The model under review builds one solid part; all positions refer to its coordinate system, in mm. Coordinates: 2 decimals unless noted, no trailing zeros. Write each loop counter-clockwise with the first axis right and the second up, starting at its lowest first coordinate (ties: lowest second). Pieces come first, ordered by that corner, then holes. Notation, with made-up numbers: (-29.5, -1.5) - (-17.5, -1.5) arc R10 cw to (-17.5, 5.5) - close; hole circle Ø6 at (67, 49). An arc over 180 degrees is marked (long way). Use one line per item in the form item = value. Start each with the question number.
```python
from build123d import *

# Parameters (mm, degrees)
SKETCH1_R           = 1.6
SKETCH1_R_2         = 3
BOSS_EXTRUDE1_DEPTH = 4
SKETCH2_R           = 11.550203763
CUT_EXTRUDE1_DEPTH  = 5


with BuildPart() as part:
    # Sketch1 → Boss-Extrude1 (new body)
    with BuildSketch(Plane.XY):
        with BuildLine():
            Line((27.071068699, -55.594908829), (62.571068699, -55.594908829))
            Line((62.571068699, -55.594908829), (62.571068699, -100.594908829))
            Line((62.571068699, -100.594908829), (24.071068699, -100.594908829))
            Line((24.071068699, -100.594908829), (24.071068699, -58.594908829))
            ThreePointArc((24.071068699, -58.594908829), (24.949748355, -56.473588486), (27.071068699, -55.594908829))
        make_face()
        with Locations((28.571068699, -64.094908829)):
            Circle(SKETCH1_R, mode=Mode.SUBTRACT)
        with Locations((44.071068699, -79.594908829)):
            Circle(SKETCH1_R_2, mode=Mode.SUBTRACT)
        with Locations((59.571068699, -64.094908829)):
            Circle(SKETCH1_R, mode=Mode.SUBTRACT)
        with Locations((28.571068699, -95.094908829)):
            Circle(SKETCH1_R, mode=Mode.SUBTRACT)
        with Locations((59.571068699, -95.094908829)):
            Circle(SKETCH1_R, mode=Mode.SUBTRACT)
    extrude(amount=BOSS_EXTRUDE1_DEPTH)

    # Sketch2 → Cut-Extrude1 (cut)
    with BuildSketch(Plane(origin=(0, 0, 0), x_dir=(-1, 0, 0), z_dir=(0, 0, -1))):
        with Locations((-44.071068699, -79.594908829)):
            Circle(SKETCH2_R)
    extrude(amount=-CUT_EXTRUDE1_DEPTH, mode=Mode.SUBTRACT)


solid = part.part
```
1. Take a section at B-B (x = 40.5). State the section outline as (y, z) points.
2. Take a section at A-A (y = -84.5). State the section outline as (x, z) points, plus the area to 3 significant figures.
3. Take a section at D-D (x = 60.5). State the section outline as (y, z) points, plus the area to 3 significant figures.
4. For L1, parallel to X at y = -64, z = 3.6; L2, parallel to Y at x = 44, z = 3.75; L3, parallel to Y at x = 44.5, z = 0.75, list the stretches that pass through material, from the lowest coordinate up.
5. The part is to be moulded in two halves that separate along X. For faces 1 (the cylindrical face through (24.927, -56.497, 1.972)), 2 (the cylindrical face through (38.74, -89.84, 1.97)), 3 (the cylindrical face through (58.392, -94.014, 1.972)), 4 (the flat face through (45, -55.595, 2)), say which applies: released by +X, released by -X, zero draft, split by the parting line, or undercut.
6. Take a section at C-C (z = 0.8). State the section outline as (x, y) points.
Returned:
q1.outline = (-100.59, 0) - (-90.58, 0) - (-90.58, 4) - (-100.59, 4) - close; (-68.61, 0) - (-55.59, 0) - (-55.59, 4) - (-68.61, 4) - close
q2.outline = (24.07, 0) - (33.61, 0) - (33.61, 4) - (24.07, 4) - close; (54.53, 0) - (62.57, 0) - (62.57, 4) - (54.53, 4) - close
q2.area = 70.3 mm²
q3.outline = (-100.59, 0) - (-96.4, 0) - (-96.4, 4) - (-100.59, 4) - close; (-93.79, 0) - (-65.4, 0) - (-65.4, 4) - (-93.79, 4) - close; (-62.79, 0) - (-55.59, 0) - (-55.59, 4) - (-62.79, 4) - close
q3.area = 159 mm²
q4.L1 = 24.07 to 26.97, 30.17 to 57.97, 61.17 to 62.57
q4.L2 = -100.59 to -91.14, -68.04 to -55.59
q4.L3 = -100.59 to -91.14, -68.05 to -55.59
q5.face_1 = released by -X
q5.face_2 = undercut
q5.face_3 = undercut
q5.face_4 = zero draft
q6.outline = (24.07, -100.59) - (62.57, -100.59) - (62.57, -55.59) - (27.07, -55.59) arc R3 ccw to (24.07, -58.59) - close; hole circle Ø3.2 at (28.57, -95.09); hole circle Ø3.2 at (28.57, -64.09); hole circle Ø23.1 at (44.07, -79.59); hole circle Ø3.2 at (59.57, -95.09); hole circle Ø3.2 at (59.57, -64.09)
